Autodesk Inventor part; units mm, degrees
ref_plane "YZ Plane" through (0, 0, 0) normal (1, 0, 0) x (0, 1, 0)
ref_plane "XZ Plane" through (0, 0, 0) normal (0, 1, 0) x (-1, 0, 0)
ref_plane "XY Plane" through (0, 0, 0) normal (0, 0, 1) x (1, 0, 0)
sketch "Sketch1" plane through (0, 0, 0) normal (0, 1, 0) x (-1, 0, 0)
  line L0 (-30, -30) -> (30, -30)
  line L1 (30, -30) -> (30, 30)
  line L2 (30, 30) -> (-30, 30)
  line L3 (-30, 30) -> (-30, -30)
  line L4 (-30, -30) -> (30, 30) construction
  line L5 (30, -30) -> (-30, 30) construction
  circle A0 centre (0, 0) radius 7.5
  circle A1 centre (-25, 25) radius 1.95
  circle A2 centre (0, 25) radius 1.95
  circle A3 centre (0, 25) radius 1.95
  circle A4 centre (25, 0) radius 1.95
  circle A5 centre (25, -25) radius 1.95
  circle A6 centre (-25, 25) radius 1.95
  circle A7 centre (-25, -25) radius 1.95
  circle A8 centre (25, 25) radius 1.95
  circle A9 centre (-25, 0) radius 1.95
  circle A10 centre (0, -25) radius 1.95
  line L6 (28, 30) -> (30, 28)
  line L7 (30, 28) -> (30, -28)
  line L8 (30, -28) -> (28, -30)
  line L9 (28, -30) -> (-28, -30)
  line L10 (-28, -30) -> (-30, -28)
  line L11 (-30, -28) -> (-30, 28)
  line L12 (-30, 28) -> (-28, 30)
  line L13 (-28, 30) -> (28, 30)
  dimension "d0" = 60
  dimension "d1" = 60
  dimension "d13" = 15
extrude "Extrusion1" add sketch "Sketch1" along normal blind 8 contours L3 L10 L0 | L10 L3 L12 L2 L6 L1 L8 L0 | L8 L1 L0 | L3 L2 L12 | L6 L2 L1 | A1 | A2 | A4 | A5 | A7 | A8 | A9 | A10
sketch "Sketch2" plane through (0, 8, 0) normal (0, 1, 0) x (1, 0, 0)
  line L0 (30, 30) -> (-30, 30)
  line L1 (-30, 30) -> (-30, -30)
  line L2 (-30, -30) -> (30, -30)
  line L3 (30, -30) -> (30, 30)
  line L4 (17.5, -17.5) -> (-17.5, -17.5)
  line L5 (-17.5, -17.5) -> (-17.5, 17.5)
  line L6 (-17.5, 17.5) -> (17.5, 17.5)
  line L7 (17.5, 17.5) -> (17.5, -17.5)
  line L8 (17.5, -17.5) -> (-17.5, 17.5) construction
  line L9 (-17.5, -17.5) -> (17.5, 17.5) construction
  line L10 (0, -17.5) -> (0, 17.5)
  line L11 (-17.5, 0) -> (17.5, 0)
  point P0 (0, 0)
  dimension "d4" = 35
  dimension "d5" = 35
hole "Hole1" at (-17.5, 8, 17.5) at (-17.5, 8, -17.5) at (17.5, 8, -17.5) at (17.5, 8, 17.5) direction (0, -1, 0) diameter 3.9 depth 10 tip angle 118
chamfer "Chamfer1" distance 2 angle 45 4 edges at (30, 4, 30) (30, 4, -30) (-30, 4, -30) (-30, 4, 30)
sketch "Sketch3" plane through (0, 8, 0) normal (0, 1, 0) x (1, 0, 0)
  line L0 (-28, -30) -> (-30, -28)
  line L1 (-28, -30) -> (28, -30)
  line L2 (30, -28) -> (28, -30)
  line L3 (30, -28) -> (30, 28)
  line L4 (28, 30) -> (30, 28)
  line L5 (28, 30) -> (-28, 30)
  line L6 (-30, 28) -> (-28, 30)
  line L7 (-30, 28) -> (-30, -28)
  circle A0 centre (17.5, 17.5) radius 1.95
  circle A1 centre (-17.5, -17.5) radius 1.95
  circle A2 centre (-17.5, 17.5) radius 1.95
  circle A3 centre (17.5, -17.5) radius 1.95
  circle A4 centre (0, 0) radius 7.5
  line L8 (25, -25) -> (-25, -25)
  line L9 (-25, -25) -> (-25, 25)
  line L10 (-25, 25) -> (25, 25)
  line L11 (25, 25) -> (25, -25)
  line L12 (25, -25) -> (-25, 25) construction
  line L13 (-25, -25) -> (25, 25) construction
  dimension "d17" = 50
  dimension "d18" = 50
hole "Hole2" at (-25, 8, -25) at (25, 8, -25) at (25, 8, 25) at (-25, 8, 25) direction (0, -1, 0) diameter 4.65 end through all
sketch "Sketch4" plane through (30, 0, 28) normal (1, 0, 0) x (0, 0, -1)
  line L0 (56, 8) -> (56, 0)
  line L1 (0, 8) -> (56, 8)
  line L2 (0, 0) -> (0, 8)
  line L3 (0, 0) -> (56, 0)
  circle A0 centre (28, 4) radius 1.5
  line L4 (-2, 8) -> (-2, 0)
  point P0 (28, 0)
  dimension "d26" = 3
  dimension "d27" = 4
  dimension "d28" = 30
extrude "Extrusion2" cut sketch "Sketch4" against normal through all contours A0
sketch "Sketch5" plane through (0, 8, 0) normal (0, 1, 0) x (1, 0, 0)
  circle A0 centre (25, -25) radius 2.325
  circle A1 centre (-25, -25) radius 2.325
  circle A2 centre (25, 25) radius 2.325
  circle A3 centre (-25, 25) radius 2.325
  circle A4 centre (10, -25) radius 1.45
  circle A5 centre (-10, -25) radius 1.45
  circle A6 centre (10, 25) radius 1.45
  circle A7 centre (-10, 25) radius 1.45
  point P0 (0, 0)
  dimension "d31" = 2.9
  dimension "d32" = 2.9
  dimension "d33" = 15
  dimension "d34" = 15
  dimension "d35" = 2.9
  dimension "d36" = 2.9
extrude "Extrusion3" cut sketch "Sketch5" against normal blind 10 contours A4 | A5 | A6 | A7
pattern_circular "Circular Pattern1" count 2 over 90 about axis through (0, 0, 0) along (0, 1, 0) of "Extrusion3"
properties part number "00_XY_stage-CHUO_SEIKI_LD-647-R1-Top"
CAD build for the part. Positions are in the model's coordinates, mm. Give positions to 0.01 mm unless a question says otherwise; leave off trailing zeros. Order: outer loops, then holes, each group sorted by start corner. A loop starts at its lowest first (then second) coordinate and runs counter-clockwise, first axis right, second up.
(1) Saw through at D-D, the plane z = 0. Give the cut face in (x, y), then the cut area to 3 significant figures.
(2) Drill centre lines: L1, parallel to X at y = 1.75, z = 25 (3 decimals); L2, parallel to X at y = 4, z = -17.5; L3, parallel to X at y = 3.75, z = -10. Where is each one in solid material? Low to high.
(3) Mould opens along X. For faces 1 (the flat face through (7, 8, 7)), 2 (the cylindrical face through (23.429, 3.944, 23.286)), 3 (the flat face through (29, 4, 29)) say: released by +X, released by -X, zero draft, split by the parting line, or undercut.
(4) Flat gauge pins, fed straight in: pin 1 (3.5 mm diameter, centred on x = -10, z = 25, fed in from -Y); pin 2 (3 mm diameter, centred on x = -17.5, z = 17.5, fed in from +Y). Where does each tip first touch, or does it go through?
(5) Saw through at A-A, the plane y = 4. State how many separate pieces and enclosed holes the cut face has, then the cut area to 3 significant figures.
(6) Saw through at B-B, the plane x = 0. Give the cut face in (y, z), then the cut area to 3 significant figures.
(7) Saw through at C-C, the plane z = -25. Give the cut face in (x, y) (3 decimals).
Results found:
1. outline: (-30, 0) - (-7.5, 0) - (-7.5, 2.5) - (-30, 2.5) - close; (-30, 5.5) - (-7.5, 5.5) - (-7.5, 8) - (-30, 8) - close; (7.5, 0) - (30, 0) - (30, 2.5) - (7.5, 2.5) - close; (7.5, 5.5) - (30, 5.5) - (30, 8) - (7.5, 8) - close
1. area: 225 mm2
2. L1: x = -30 to -27.325, -22.675 to -11.45, -8.55 to 8.55, 11.45 to 22.675, 27.325 to 30
2. L2: x = -30 to -19.45, -15.55 to 15.55, 19.45 to 30
2. L3: x = -30 to -26.45, -23.55 to 23.55, 26.45 to 30
3. face 1: zero draft
3. face 2: undercut
3. face 3: released by +X
4. pin 1: stops at y = 0
4. pin 2: passes through
5. separate pieces: 2
5. enclosed holes: 16
5. area: 3,110 mm2
6. outline: (0, -30) - (8, -30) - (8, -7.5) - (0, -7.5) - close; (0, 7.5) - (8, 7.5) - (8, 30) - (0, 30) - close
6. area: 360 mm2
7. outline: (-30, 0) - (-27.325, 0) - (-27.325, 8) - (-30, 8) - close; (-22.675, 0) - (-11.45, 0) - (-11.45, 8) - (-22.675, 8) - close; (-8.55, 0) - (8.55, 0) - (8.55, 8) - (-8.55, 8) - close; (11.45, 0) - (22.675, 0) - (22.675, 8) - (11.45, 8) - close; (27.325, 0) - (30, 0) - (30, 8) - (27.325, 8) - close
